Verification items for this drawing (mm, ordinates from the low corner). A direction names the side the tool comes from. Coordinates: 2 decimals unless noted, no trailing zeros. Order: outer loops, then holes, each group sorted by start corner. A loop starts at its lowest first (then second) coordinate and runs counter-clockwise, first axis right, second up. Notation, with made-up numbers: M -10,8 L 2,8 A22 cw 2,47 Z; hole C 57,58 d11. An arc over 180 degrees is marked long. One line per item, written item: value. Start each with the question number.
1) Sectioned sample at B-B, the plane z = 24.5. Enter the section's corners in (x, y).
2) Access from +Z, -Z, +X, -X, +Y, -Y to the whole of each face (thin tool, end or side, straight path). Record for the marked faces 1, 2 and 3.
3) Sectioned sample at C-C, the plane z = 16.5. Enter the section's corners in (x, y).
4) Sectioned sample at A-A, the plane y = 18. Enter the section's corners in (x, z).
5) Thickness scan on L1, parallel to X at y = 2.3, z = 24.5; L2, parallel to Y at x = 15, z = 16.05; L3, parallel to Y at x = 16, z = 8. Record the ranges inside material, lowest first. Write a range as from..to.
6) Draft check along X on the marked faces 4, 5, 6 and 7. Enter one of: pulls with the +X half, pulls with the -X half, needs draft (parallel to the pull), parting line crosses it, or undercut.
7) Sectioned sample at D-D, the plane x = 11.25. Enter the section's corners in (y, z) (1 decimal).
8) Go/stop test with flat-tipped pins: P1, Ø12, axis at x = 6.5, y = 14.5, coming from the +Z side; P2, Ø10, axis at x = 8.5, z = 9, coming from the -Y side; P3, Ø3.5, axis at x = 21.5, z = 26.5, coming from the +Y side; P4, Ø8, axis at x = 15, y = 18, coming from the -Z side. Record where each tip stops, or that it passes through.
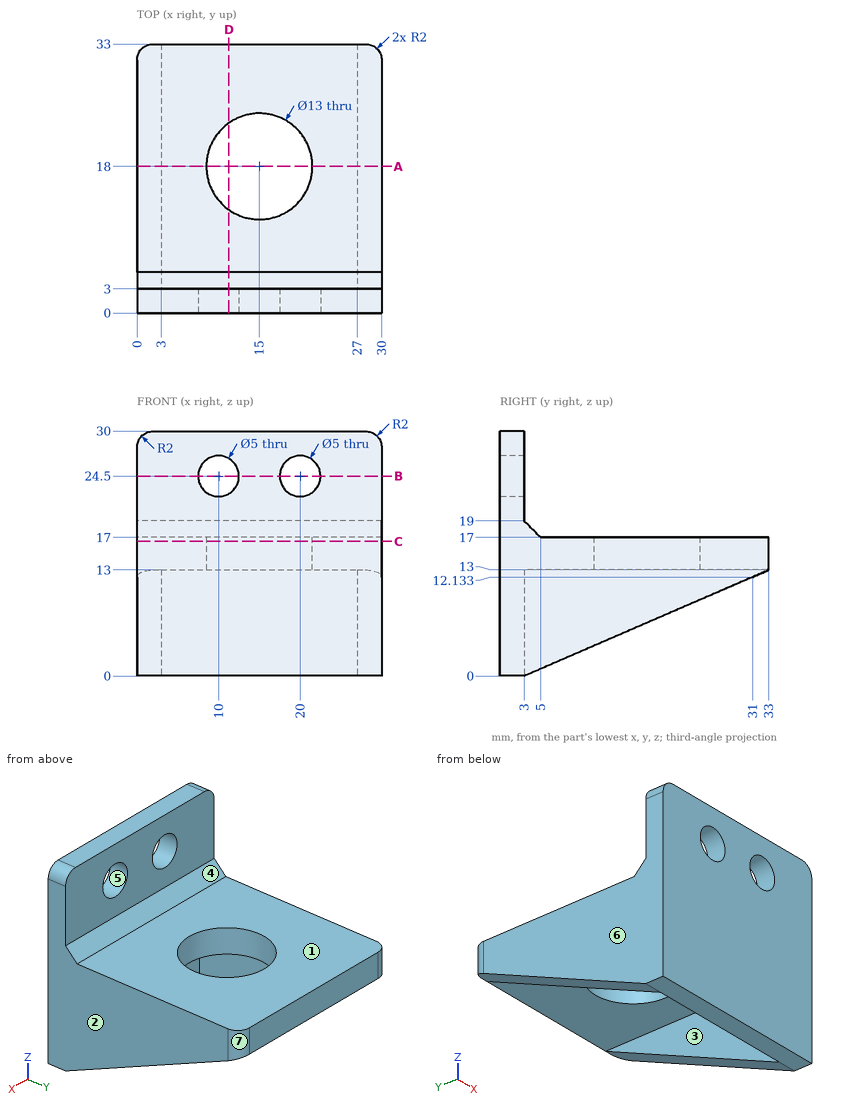
Final values:
1. outline: M 0,0 L 7.5,0 L 7.5,3 L 0,3 Z; M 12.5,0 L 17.5,0 L 17.5,3 L 12.5,3 Z; M 22.5,0 L 30,0 L 30,3 L 22.5,3 Z
2. face 1: +Z, +X, -X, +Y
2. face 2: +Z, -Z, +X, +Y, -Y
2. face 3: -Z, +Y
3. outline: M 0,0 L 30,0 L 30,31 A2 ccw 28,33 L 2,33 A2 ccw 0,31 Z; hole C 15,18 d13
4. outline: M 0,6.5 L 3,6.5 L 3,13 L 8.5,13 L 8.5,17 L 0,17 Z; M 21.5,13 L 27,13 L 27,6.5 L 30,6.5 L 30,17 L 21.5,17 Z
5. L1: x = 0..7.5, 12.5..17.5, 22.5..30
5. L2: y = 0..11.5, 24.5..33
5. L3: y = 0..3
6. face 4: needs draft
6. face 5: undercut
6. face 6: pulls with the -X half
6. face 7: pulls with the +X half
7. outline: M 0,0 L 3,0 L 3,13 L 12.7,13 L 12.7,17 L 5,17 L 3,19 L 3,22.3 L 0,22.3 Z; M 0,26.7 L 3,26.7 L 3,30 L 0,30 Z; M 23.3,13 L 33,13 L 33,17 L 23.3,17 Z
8. P1: stops at z = 17
8. P2: stops at y = 0
8. P3: stops at y = 3
8. P4: passes through
